from build123d import *

# Parameters (mm, degrees)
SKETCH2_W          = 6
SKETCH2_H          = 7
CUT_EXTRUDE1_DEPTH = 41.4
SKETCH3_R          = 2
CUT_EXTRUDE2_DEPTH = 29
SKETCH4_R          = 2
CUT_EXTRUDE3_DEPTH = 29


with BuildPart() as part:
    # Sketch1 → Revolve1 (revolve)
    with BuildSketch(Plane.XY, mode=Mode.PRIVATE) as revolve1_sk:
        Polygon((11, 0), (11, 41.4), (3.25, 41.4), (3.25, 49.8), (6, 49.8), (6, 57.8), (22.825, 57.8), (22.825, 45.8), (17.5, 45.8), (17.5, 22.9), (21.45, 19.3), (21.45, 12), (22.5, 11.3), (22.5, 0.8), (21.75, 0), align=None)
    revolve(revolve1_sk.sketch.rotate(Axis((0, 0, 0), (0, 1, 0)), 90), axis=Axis((0, 0, 0), (0, 1, 0)))

    # Sketch2 → Cut-Extrude1 (cut)
    with BuildSketch(Plane.XZ):
        with Locations((0, 10.5)):
            Rectangle(SKETCH2_W, SKETCH2_H)
    extrude(amount=-CUT_EXTRUDE1_DEPTH, mode=Mode.SUBTRACT)

    # Sketch3 → Cut-Extrude2 (cut)
    with BuildSketch(Plane.XY.offset(22)):
        with Locations((0, 16.5)):
            Circle(SKETCH3_R)
    extrude(amount=-CUT_EXTRUDE2_DEPTH, mode=Mode.SUBTRACT)

    # Sketch4 → Cut-Extrude3 (cut)
    with BuildSketch(Plane(origin=(22, 0, 0), x_dir=(0, 0, -1), z_dir=(1, 0, 0))):
        with Locations((0, 16.5)):
            Circle(SKETCH4_R)
    extrude(amount=-CUT_EXTRUDE3_DEPTH, mode=Mode.SUBTRACT)


solid = part.part
The listing builds one solid part. Answer for the finished solid, in the listing's coordinates (mm). A direction names the side the tool comes from. Give positions to 0.01 mm unless a question says otherwise; leave off trailing zeros. Write each loop counter-clockwise with the first axis right and the second up, starting at its lowest first coordinate (ties: lowest second). Pieces come first, ordered by that corner, then holes.
Item 1: Flat-ended cylindrical pins translate along their axes: P1, Ø6, axis at x = -9.5, y = 23, coming from the -Z side; P2, Ø9.5, axis at x = -0.5, z = 0.5, coming from the +Y side; P3, Ø2.5, axis at y = 22, z = 12, coming from the +X side; P4, Ø10, axis at x = -4, z = -7.5, coming from the -Y side. Find the tip coordinate at first contact, or state that the pin passes through.
Item 2: Section A-A, the plane x = 0 is taken. Count the separate pieces of the cut face and the enclosed holes in it, plus the area to 3 significant figures.
Item 3: Which of the six approach directions +Z, -Z, +X, -X, +Y, -Y give full straight-line access (tool end or side, diameter ignored) to faces 4 (the cylindrical face through (-0.26, 18.483, 17.778)), 5 (the cylindrical face through (19.961, 5.977, -10.382)), 6 (the cylindrical face through (16.206, 18.483, 0.26)), 7 (the flat face through (17, 45.8, 5)), 8 (the cylindrical face through (-1.802, 53.856, -5.723))?
Item 4: Determine the mould class of faces 1 (the cylindrical face through (0, 21, -11)), 2 (the cylindrical face through (17.084, 34.19, 3.794)), 3 (the flat face through (-5, 0, 10)) for opening direction X: released by +X, released by -X, zero draft, split by the parting line, or undercut.
Item 5: Find the intervals of material crossed by line 1 along Y through (x, z) = (-1.5, 19.5); line 2 along X through (y, z) = (44, 0); line 3 along X through (y, z) = (46.25, 0) (3 decimals), in increasing order.
Item 6: Section C-C, the plane y = 20 is taken. Write down the section's boundary in (x, z).
Completed:
1. P1: stops at z = -18.65
1. P2: stops at y = 49.8
1. P3: stops at x = 16.06
1. P4: stops at y = 0
2. separate pieces: 3
2. enclosed holes: 0
2. area: 1,130 mm2
3. face 4: +Z
3. face 5: -Y
3. face 6: +X
3. face 7: none
3. face 8: +Y
4. face 1: undercut
4. face 2: split by the parting line
4. face 3: zero draft
5. line 1: y = 0 to 15.18, 17.82 to 21.02, 45.8 to 57.8
5. line 2: x = -17.5 to -3.25, 3.25 to 17.5
5. line 3: x = -22.825 to -3.25, 3.25 to 22.825
6. outline: circle Ø41.36 at (0, 0); hole (-3, 10.58) arc R11 ccw (long way) to (3, 10.58) - (3, 14) - (-3, 14) - close
